Verification items for this drawing (mm, ordinates from the low corner). Give positions to 0.01 mm unless a question says otherwise; leave off trailing zeros. Order: outer loops, then holes, each group sorted by start corner. A loop starts at its lowest first (then second) coordinate and runs counter-clockwise, first axis right, second up. Notation, with made-up numbers: M 33,66 L 72,66 A10 ccw 72,73 Z; hole C 35,11.5 d1. An arc over 180 degrees is marked long. Answer as a JSON object with one key per item and string values.
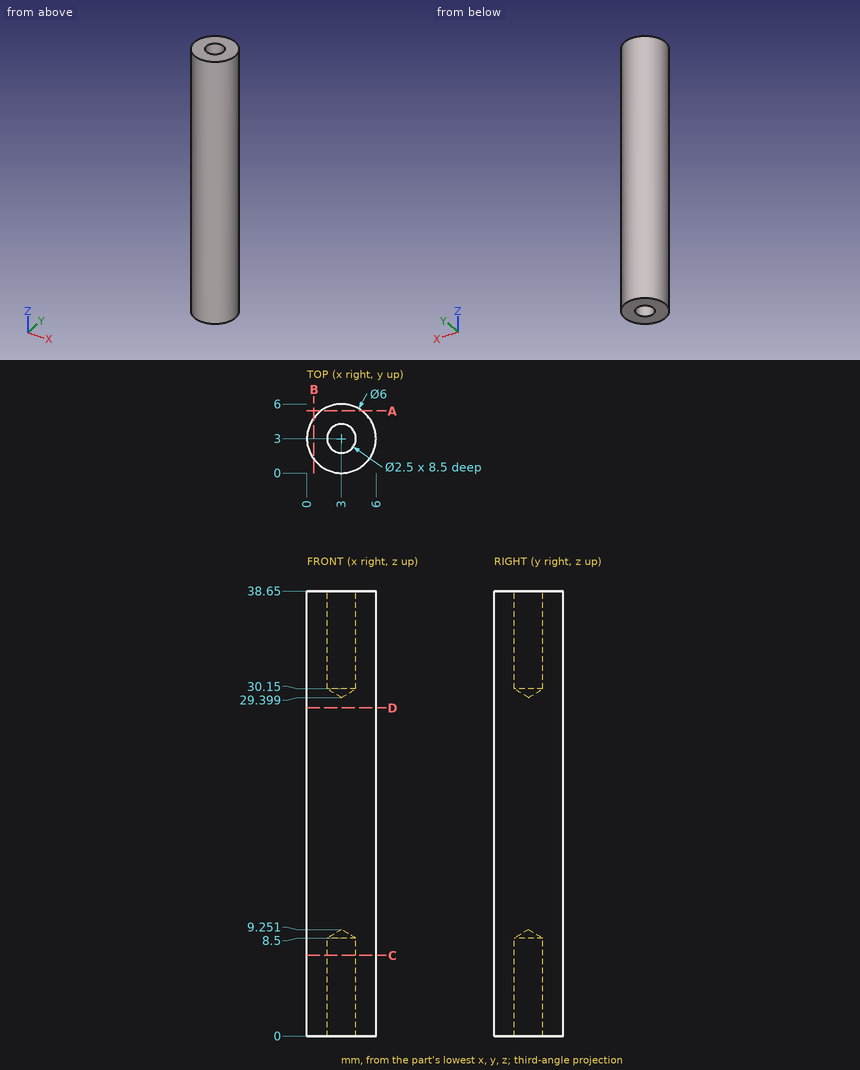
Q1. Section check A-A on y = 5.4. Record the cut outline in (x, z).
Resolved:
{"outline": "M 1.2,0 L 4.8,0 L 4.8,38.65 L 1.2,38.65 Z"}
Q2. Gauge pin test, flat end, axial feed: pin 1 Ø3 at (y, z) = (1.5, 17.5) entering from +X. Record the tip position at first contact, or that the pin passes through.
Resolved:
{"pin 1": "stops at x = 6"}
Q3. Section check D-D on z = 28.5. Record the cut outline in (x, y), then the cut area to 3 significant figures.
Resolved:
{"outline": "C 3,3 d6", "area": "28.3 mm²"}
Q4. Material ranges on L1, parallel to Y at x = 3, z = 4.25; L2, parallel to X at y = 1.9, z = 3; L3, parallel to X at y = 2.9, z = 19, recorded low to high.
Resolved:
{"L1": "y = 0 to 1.75, 4.25 to 6", "L2": "x = 0.21 to 2.41, 3.59 to 5.79", "L3": "x = 0 to 6"}
Q5. Section check C-C on z = 7. Record the cut outline in (x, y), then the cut area to 3 significant figures.
Resolved:
{"outline": "C 3,3 d6; hole C 3,3 d2.5", "area": "23.4 mm²"}
